Read the model definition and answer for the solid it produces. Units are mm, in the model's axes. Round coordinates to 2 decimals unless told otherwise and drop trailing zeros. Write each loop counter-clockwise with the first axis right and the second up, starting at its lowest first coordinate (ties: lowest second). Pieces come first, ordered by that corner, then holes. Notation, with made-up numbers: (-8, 45.5) -> (24, 45.5) arc R33 ccw to (24, 80.5) -> close; hole circle Ø7 at (72.5, -11.5). An arc over 180 degrees is marked (long way). Return JSON: item names as keys, results as strings. Group by question number.
(1) Straight lines are drawn through the part: line 1 (Z direction, x = 130.5, y = -444.5); line 2 (X direction, y = -388, z = 303.5); line 3 (X direction, y = -520, z = 211). For each, find the intervals that lie inside material, in ascending order.
(2) Given pin 1 (4 mm diameter, centred on x = 114.5, z = 400, fed in from +Y); pin 2 (12 mm diameter, centred on x = 159, z = 324.5, fed in from -Y); pin 3 (1 mm diameter, centred on x = 198.5, z = 346, fed in from +Y), each flat-ended and moving along its own axis, determine where each tip first touches the part or whether it passes through.
(3) A cutting plane is placed at A-A on z = 246.5. Give the vertices of the cut face in (x, y).
(4) A cutting plane is placed at B-B on y = -518. Give the vertices of the cut face in (x, z).
```python
from build123d import *

# Parameters (mm, degrees)
PAD002_DEPTH = 600
FILLET002_R  = 124
FILLET003_R  = 25


with BuildPart() as part:
    # Sketch002 → Pad002 (new body)
    with BuildSketch(Plane.XZ):
        with BuildLine():
            Line((0, 0), (250, 0))
            Line((250, 0), (250, 100))
            ThreePointArc((250, 100), (125, 225), (0, 100))
            Line((0, 100), (0, 0))
        make_face()
    extrude(amount=PAD002_DEPTH)

    # Fillet002
    fillet002_edges = [part.edges().sort_by_distance(p)[0] for p in [
        (125, 0, 225),
        (125, -600, 225),
    ]]
    fillet(fillet002_edges, radius=FILLET002_R)

    # Fillet003
    fillet003_edges = [part.edges().sort_by_distance(p)[0] for p in [
        (0, -300, 0),
        (36.318759, -36.318759, 0),
        (36.318759, -563.681241, 0),
        (125, 0, 0),
        (125, -600, 0),
        (213.681241, -36.318759, 0),
        (213.681241, -563.681241, 0),
        (250, -300, 0),
        (0, -300, 100),
        (0, -124, 50),
        (0, -476, 50),
        (36.318759, -36.318759, 100),
        (124, 0, 50),
        (36.318759, -563.681241, 100),
        (124, -600, 50),
        (126, 0, 50),
        (125, 0, 101),
        (126, -600, 50),
        (125, -600, 101),
        (250, -124, 50),
        (213.681241, -36.318759, 100),
        (250, -476, 50),
        (213.681241, -563.681241, 100),
        (250, -300, 100),
        (125, -124, 225),
        (125, -476, 225),
    ]]
    fillet(fillet003_edges, radius=FILLET003_R)


with BuildPart() as part_1:
    # Body002 placement: moved
    add(part.part.moved(Location((0, -100, 200))))


solid = part_1.part
```
Checks:
{
 "1": {"line 1": "z = 200 to 424.88", "line 2": "x = 0.05 to 249.95", "line 3": "x = 4.29 to 245.71"},
 "2": {"pin 1": "stops at y = -147.45", "pin 2": "stops at y = -694.99", "pin 3": "stops at y = -133.91"},
 "3": {"outline": "(0, -576) arc R124 ccw to (124, -700) -> (126, -700) arc R124 ccw to (250, -576) -> (250, -224) arc R124 ccw to (126, -100) -> (124, -100) arc R124 ccw to (0, -224) -> close"},
 "4": {"outline": "(0, 225) arc R25 ccw to (25, 200) -> (225, 200) arc R25 ccw to (250, 225) -> (250, 300) arc R125 ccw to (0, 300) -> close"}
}
